Read the model definition and answer for the solid it produces. Units are mm, in the model's axes. A direction names the side the tool comes from. Coordinates: 2 decimals unless noted, no trailing zeros. Order: outer loops, then holes, each group sorted by start corner. A loop starts at its lowest first (then second) coordinate and runs counter-clockwise, first axis right, second up. Notation, with made-up numbers: M 40.5,-28.5 L 60.5,-28.5 A9 cw 60.5,-15.5 Z; hole C 84,6.5 d7. An arc over 180 degrees is marked long. One line per question, with ' | ' between items. Start each with the question number.
1) Given P1, Ø5, axis at y = 37, z = 4.5, coming from the +X side; P2, Ø2, axis at x = -34.5, y = -3.5, coming from the -Z side; P3, Ø10, axis at x = -30.5, y = 44, coming from the +Z side; P4, Ø9.5, axis at x = -26, y = 28, coming from the +Z side, each flat-ended and moving along its own axis, determine where each tip first touches the part or whether it passes through.
2) Find section A-A, the plane z = 10. Write down the section's boundary in (x, y), plus the area to 3 significant figures.
3) A tool of negligible diameter and unlimited length cuts with its end or side. For faces 1 (the face through (-35, 52.011, 4)), 2 (the face through (-33.971, 23, 15)), 3 (the face through (-35, -2.989, 18)), 4 (the face through (-35, -4, 5)), from which of +Z, -Z, +X, -X, +Y, -Y can it reach the whole face along a straight path? Write none if from no direction.
4) The mould has two halves that part along Y. Classify faces 5 (the face through (-35, 25, 20)), 6 (the face through (-27, -2.989, -1)), 7 (the face through (-34.985, 46.225, 9.447)): +Y half, -Y half, draft (parallel to the pull), parting line (faces both ways), or undercut.
5) Find section D-D, the plane z = 7. Write down the section's boundary in (x, y), plus the area to 3 significant figures.
6) Find section B-B, the plane y = 19. Write down the section's boundary in (x, z).
7) Find section C-C, the plane y = 9. Write down the section's boundary in (x, z), plus the area to 3 significant figures.
8) Consider probe 1 along Y at (x, z) = (-34.75, 10); probe 2 along X at (y, z) = (29, 7.75); probe 3 along Z at (x, y) = (-28.5, 37.5). Determine where each line is inside the solid, lowest interval first.
from build123d import *

# Parameters (mm, degrees)
SKETCH_1_W                       = 2
SKETCH_1_H                       = 55
SM_BASE_FLANGE_1_DEPTH           = 20
SM_EDGE_FLANGE_1_STRIP_W         = 10.4
SM_EDGE_FLANGE_1_STRIP_H         = 2
SM_EDGE_FLANGE_1_STRIP_CUT_DEPTH = 55
SM_EDGE_FLANGE_1_DEPTH           = 55
SKETCH_6_W                       = 2
SKETCH_6_H                       = 10
EXTRUDE_1_DEPTH                  = 2
SKETCH_8_R                       = 4.25
CUT_EXTRUDE_2_DEPTH              = 5


# Sheet-metal steps are written as plain solids
with BuildPart() as part:
    # Sketch 1 → Базовая кромка1 (new body)
    with BuildSketch(Plane.XY):
        with Locations((-34.970714213, 24.511351052)):
            Rectangle(SKETCH_1_W, SKETCH_1_H)
    extrude(amount=SM_BASE_FLANGE_1_DEPTH)

    # Ребро-кромка1 strip (across the edge) → Ребро-кромка1 strip cut (cut)
    with BuildSketch(Plane(origin=(-33.970714213, -2.988648948, 0), x_dir=(0, 0, 1), z_dir=(0, 1, 0))):
        with Locations((-4, -1)):
            Rectangle(SM_EDGE_FLANGE_1_STRIP_W, SM_EDGE_FLANGE_1_STRIP_H)
    extrude(amount=SM_EDGE_FLANGE_1_STRIP_CUT_DEPTH, mode=Mode.SUBTRACT)

    # Ребро-кромка1 section (across the edge) → Ребро-кромка1 (add)
    with BuildSketch(Plane(origin=(-33.970714213, -2.988648948, 0), x_dir=(0, 0, 1), z_dir=(0, 1, 0))):
        with BuildLine():
            Line((-2, 1.2), (-2, 20))
            Line((-2, 20), (0, 20))
            Line((0, 20), (0, 1.2))
            ThreePointArc((0, 1.2), (0.351471863, 0.351471863), (1.2, 0))
            Line((1.2, 0), (1.2, -2))
            ThreePointArc((1.2, -2), (-1.0627417, -1.0627417), (-2, 1.2))
        make_face()
    extrude(amount=SM_EDGE_FLANGE_1_DEPTH)

    # Эскиз6 → Бобышка-Вытянуть1 (add)
    with BuildSketch(Plane.XZ.offset(2.988648948)):
        with Locations((-34.970714213, 10)):
            Rectangle(SKETCH_6_W, SKETCH_6_H)
    extrude(amount=EXTRUDE_1_DEPTH)

    # Эскиз8 → Вырез-Вытянуть2 (cut)
    with BuildSketch(Plane.ZY.offset(35.970714213)):
        with Locations((10, 42.011351052)):
            Circle(SKETCH_8_R)
        with Locations((10, 21.011351052)):
            Circle(SKETCH_8_R)
    extrude(amount=-CUT_EXTRUDE_2_DEPTH, mode=Mode.SUBTRACT)


solid = part.part
Report:
1) P1: stops at x = -33.97 | P2: stops at z = -1.88 | P3: stops at z = 20 | P4: stops at z = 0
2) outline: M -35.97,-4.99 L -33.97,-4.99 L -33.97,16.76 L -35.97,16.76 Z; M -35.97,25.26 L -33.97,25.26 L -33.97,37.76 L -35.97,37.76 Z; M -35.97,46.26 L -33.97,46.26 L -33.97,52.01 L -35.97,52.01 Z | area: 80.0 mm^2
3) face 1: +Z, -Z, +X, -X, +Y | face 2: +Z, +X, +Y, -Y | face 3: +Z, +X, -X, -Y | face 4: -Z, +X, -X, -Y
4) face 5: draft | face 6: -Y half | face 7: undercut
5) outline: M -35.97,-4.99 L -33.97,-4.99 L -33.97,18 L -35.97,18 Z; M -35.97,24.02 L -33.97,24.02 L -33.97,39 L -35.97,39 Z; M -35.97,45.02 L -33.97,45.02 L -33.97,52.01 L -35.97,52.01 Z | area: 89.9 mm^2
6) outline: M -35.97,1.2 A3.2 ccw -32.77,-2 L -13.97,-2 L -13.97,0 L -32.77,0 A1.2 cw -33.97,1.2 L -33.97,6.26 L -35.97,6.26 Z; M -35.97,13.74 L -33.97,13.74 L -33.97,20 L -35.97,20 Z
7) outline: M -35.97,1.2 A3.2 ccw -32.77,-2 L -13.97,-2 L -13.97,0 L -32.77,0 A1.2 cw -33.97,1.2 L -33.97,20 L -35.97,20 Z | area: 82.1 mm^2
8) probe 1: y = -4.99 to 16.76, 25.26 to 37.76, 46.26 to 52.01 | probe 2: x = -35.97 to -33.97 | probe 3: z = -2 to 0
